Part model, mm, in its own coordinate system. A direction names the side the tool comes from. Give positions to 0.01 mm unless a question says otherwise; leave off trailing zeros. Order: outer loops, then holes, each group sorted by start corner. A loop starts at its lowest first (then second) coordinate and runs counter-clockwise, first axis right, second up. Notation, with made-up numbers: M 8,52.25 L 29,52.25 A20 cw 29,68.25 Z; hole C -31.5,51 d10. An arc over 180 degrees is marked long. Return JSON: item names as keys, results as strings.
from build123d import *

# Parameters (mm, degrees)
BOSS_EXTRUDE4_DEPTH    = 1.6
CONVERT_SOLID6_DEPTH   = 0.6
SKETCHED_START         = -60.753452496
SKETCHED_BEND3_DEPTH   = 44
SKETCHED_BEND3_2_DEPTH = 2
SKETCHED_START_2       = -18.753452496
SKETCHED_BEND3_3_DEPTH = 2
SKETCHED_BEND3_4_DEPTH = 44
SKETCHED_START_3       = -58.753452496
SKETCHED_BEND3_5_DEPTH = 40
F_3_0MM_DOWEL_HOLE1_D  = 3
F_3_0MM_DOWEL_HOLE2_D  = 3
F_3_0MM_DOWEL_HOLE3_D  = 3
F_3_0MM_DOWEL_HOLE4_D  = 3


# Read off the part's stored shape, not the designer's step: Convert-Solid6, Sketched Bend3
with BuildPart() as part:
    # Sketch1 → Boss-Extrude4 (new body)
    with BuildSketch(Plane.XY):
        Polygon((-58.753452496, 23.769203004), (-18.753452496, 23.769203004), (-18.753452496, -16.230796996), (-16.753452496, -16.230796996), (-16.753452496, -46.230796996), (-60.753452496, -46.230796996), (-60.753452496, -16.230796996), (-58.753452496, -16.230796996), align=None)
    extrude(amount=BOSS_EXTRUDE4_DEPTH)

    # Convert-Solid6 outline → Convert-Solid6 (cut)
    with BuildSketch(Plane.XY):
        Polygon((-58.753452496, 23.769203004), (-58.753452496, -16.230796996), (-60.753452496, -16.230796996), (-60.753452496, -46.230796996), (-16.753452496, -46.230796996), (-16.753452496, -16.230796996), (-18.753452496, -16.230796996), (-18.753452496, 23.769203004), align=None)
    extrude(amount=CONVERT_SOLID6_DEPTH, mode=Mode.SUBTRACT)

    # Sketched Bend3 outline → Sketched Bend3 (cut)
    with BuildSketch(Plane.YZ.offset(SKETCHED_START)):
        with BuildLine():
            Line((-16.962847803, 1.6), (-46.230796996, 1.6))
            Line((-46.230796996, 1.6), (-46.230796996, 0.6))
            Line((-46.230796996, 0.6), (-15.230796996, 0.6))
            ThreePointArc((-15.230796996, 0.6), (-16.230796996, 0.867949193), (-16.962847803, 1.6))
        make_face()
    extrude(amount=SKETCHED_BEND3_DEPTH, mode=Mode.SUBTRACT)

    # Sketched Bend3 2 outline → Sketched Bend3 2 (cut)
    with BuildSketch(Plane.YZ.offset(SKETCHED_START)):
        with BuildLine():
            Line((-16.230796996, 1.329098256), (-16.467536602, 1.028225479))
            ThreePointArc((-16.467536602, 1.028225479), (-16.35203432, 0.9438518), (-16.230796996, 0.867949193))
            Line((-16.230796996, 0.867949193), (-16.230796996, 1.329098256))
        make_face()
    extrude(amount=SKETCHED_BEND3_2_DEPTH, mode=Mode.SUBTRACT)

    # Sketched Bend3 3 outline → Sketched Bend3 3 (cut)
    with BuildSketch(Plane.YZ.offset(SKETCHED_START_2)):
        with BuildLine():
            Line((-16.230796996, 1.329098256), (-16.467536602, 1.028225479))
            ThreePointArc((-16.467536602, 1.028225479), (-16.35203432, 0.9438518), (-16.230796996, 0.867949193))
            Line((-16.230796996, 0.867949193), (-16.230796996, 1.329098256))
        make_face()
    extrude(amount=SKETCHED_BEND3_3_DEPTH, mode=Mode.SUBTRACT)

    # Sketched Bend3 4 outline → Sketched Bend3 4 (add)
    with BuildSketch(Plane.YZ.offset(SKETCHED_START)):
        with BuildLine():
            Line((-16.230796996, 31.24380551), (-17.230796996, 31.24380551))
            Line((-17.230796996, 31.24380551), (-17.230796996, 2.6))
            ThreePointArc((-17.230796996, 2.6), (-17.162648648, 2.08236191), (-16.962847803, 1.6))
            Line((-16.962847803, 1.6), (-16.230796996, 1.6))
            Line((-16.230796996, 1.6), (-16.230796996, 1.329098256))
            Line((-16.230796996, 1.329098256), (-15.849166799, 1.814112739))
            ThreePointArc((-15.849166799, 1.814112739), (-16.130344049, 2.163176124), (-16.230796996, 2.6))
            Line((-16.230796996, 2.6), (-16.230796996, 31.24380551))
        make_face()
    extrude(amount=SKETCHED_BEND3_4_DEPTH)

    # Sketched Bend3 5 outline → Sketched Bend3 5 (add)
    with BuildSketch(Plane.YZ.offset(SKETCHED_START_3)):
        with BuildLine():
            ThreePointArc((-15.230796996, 1.6), (-15.557991693, 1.655043054), (-15.849166799, 1.814112739))
            Line((-15.849166799, 1.814112739), (-16.017639885, 1.6))
            Line((-16.017639885, 1.6), (-15.230796996, 1.6))
        make_face()
    extrude(amount=SKETCHED_BEND3_5_DEPTH)

    # Ø3.0mm Dowel Hole1 (through all)
    with Locations(Plane(origin=(-8.856923846, -7.992050606, 0.6), x_dir=(1, 0, 0), z_dir=(0, 0, -1))):
        with Locations((-43.60055999, 1.230399912)):
            Hole(F_3_0MM_DOWEL_HOLE1_D / 2)

    # Ø3.0mm Dowel Hole2 (through all)
    with Locations(Plane(origin=(-8.856923846, -7.992050606, 0.6), x_dir=(1, 0, 0), z_dir=(0, 0, -1))):
        with Locations((-17.11602881, 1.265852801)):
            Hole(F_3_0MM_DOWEL_HOLE2_D / 2)

    # Ø3.0mm Dowel Hole3 (through all)
    with Locations(Plane(origin=(-8.856923846, -7.992050606, 0.6), x_dir=(1, 0, 0), z_dir=(0, 0, -1))):
        with Locations((-43.586196393, -25.265955548)):
            Hole(F_3_0MM_DOWEL_HOLE3_D / 2)

    # Ø3.0mm Dowel Hole4 (through all)
    with Locations(Plane(origin=(-8.856923846, -7.992050606, 0.6), x_dir=(1, 0, 0), z_dir=(0, 0, -1))):
        with Locations((-17.044209907, -25.235902464)):
            Hole(F_3_0MM_DOWEL_HOLE4_D / 2)


solid = part.part
Q1. Band-saw the part on C-C (z = 7.5). Give the cut face in (x, y).
Established:
{"outline": "M -60.75,-17.23 L -16.75,-17.23 L -16.75,-16.23 L -60.75,-16.23 Z"}
Q2. Pin check, flat tips, straight feed: pin 1 (1.8 mm diameter, centred on x = -52.44, y = 17.27, fed in from +Z); pin 2 (1 mm diameter, centred on y = 8.5, z = 1.5, fed in from -X); pin 3 (0.6 mm diameter, centred on y = 7.5, z = 1.5, fed in from +X); pin 4 (8 mm diameter, centred on x = -51.5, y = 11.5, fed in from +Z). Stop position of each tip, or through.
Established:
{"pin 1": "passes through", "pin 2": "stops at x = -58.75", "pin 3": "stops at x = -18.75", "pin 4": "stops at z = 1.6"}
Q3. 3-axis set-ups, long thin cutter, end or side, ignore diameter. For faces 4 (the flat face through (-38, 5, 1.6)), 5 (the flat face through (-39, 5, 0.6)): which of +Z, -Z, +X, -X, +Y, -Y reach the whole face in a straight line?
Established:
{"face 4": "+Z, +X, -X, +Y", "face 5": "-Z, +X, -X, +Y, -Y"}
Q4. Band-saw the part on D-D (y = 20). Give the cut face in (x, z), then the cut area to 3 significant figures.
Established:
{"outline": "M -58.75,0.6 L -18.75,0.6 L -18.75,1.6 L -58.75,1.6 Z", "area": "40.0 mm²"}
Q5. Band-saw the part on B-B (x = -25.5). Give the cut face in (y, z), then the cut area to 3 significant figures.
Established:
{"outline": "M -17.23,2.6 A2 ccw -15.23,0.6 L -10.68,0.6 L -10.68,1.6 L -15.23,1.6 A1 cw -16.23,2.6 L -16.23,31.24 L -17.23,31.24 Z; M -7.83,0.6 L 15.8,0.6 L 15.8,1.6 L -7.83,1.6 Z; M 18.69,0.6 L 23.77,0.6 L 23.77,1.6 L 18.69,1.6 Z", "area": "64.3 mm²"}
Q6. Probe line 1 along Y through (x, z) = (-42.5, 22.5); line 2 along Z through (x, y) = (-53, 10). List the from-to ranges inside material, lowest first.
Established:
{"line 1": "y = -17.23 to -16.23", "line 2": "z = 0.6 to 1.6"}
Q7. Two-plate mould, pull along X, no slides. Class faces 1 (the flat face through (-18.753, 3, 1)), 2 (the cylindrical face through (-51.3, 16.3, 1.1)), 3 (the flat face through (-39, -17.231, 17)): +X half, -X half, draft (parallel to the pull), parting line (faces both ways), or undercut.
Established:
{"face 1": "+X half", "face 2": "undercut", "face 3": "draft"}
Q8. Band-saw the part on A-A (x = -40.5). Give the cut face in (y, z), then the cut area to 3 significant figures.
Established:
{"outline": "M -17.23,2.6 A2 ccw -15.23,0.6 L 23.77,0.6 L 23.77,1.6 L -15.23,1.6 A1 cw -16.23,2.6 L -16.23,31.24 L -17.23,31.24 Z", "area": "70.0 mm²"}
